Autodesk Inventor part; units mm, degrees
ref_plane "Work Plane1" through (29, 0, 0) normal (0, -1, 0) x (1, 0, 0)
ref_plane "YZ Plane" through (0, 0, 0) normal (1, 0, 0) x (0, 1, 0)
ref_plane "XZ Plane" through (0, 0, 0) normal (0, 1, 0) x (-1, 0, 0)
sketch "Sketch1" plane through (0, 0, 0) normal (0, 0, 1) x (1, 0, 0)
  line L0 (-0.0667, 0) -> (16, 0)
  line L1 (16, 0) -> (16, 2)
  line L2 (16, 2) -> (2.1, 2)
  line L3 (2.1, 2) -> (1.6705, 2)
  line L4 (1.6705, 2) -> (0, 2)
  line L5 (0, 2) -> (0, 3.8)
  line L6 (0, 3.8) -> (-2.2, 3.8)
  line L7 (-2.2, 3.8) -> (-2.2, 1.4434)
  line L8 (-2.2, 1.4434) -> (-0.9, 1.4434)
  line L9 (-0.9, 1.4434) -> (-0.0667, 0)
  line L10 (-5.84, 0) -> (19.64, 0)
  line L11 (0, -0.76) -> (0, 4.56)
  line L12 (2.1, 2) -> (0, 2) construction
  dimension "d1" = 13.9
  dimension "d2" = 0.4295
  dimension "d3" = 2.2
  dimension "d4" = 1.3
  dimension "d5" = 60
  dimension "d6" = 4
  dimension "d7" = 4
  dimension "d8" = 2.8868
  dimension "d9" = 7.6
  dimension "d26" = 16
revolve "Body" add sketch "Sketch1" angle 360 about axis through (-0.0667, 0, 0) along (1, 0, 0)
sketch "Sketch2" plane through (-2.2, 0, 0) normal (-1, 0, 0) x (0, 0, 1)
  circle A0 centre (0, 0) radius 1.4434
  line L0 (0, -5.32) -> (0, 5.32)
  line L1 (-5.32, 0) -> (5.32, 0)
  line L2 (1.4434, 0) -> (0.7217, -1.25)
  line L3 (0.7217, -1.25) -> (-0.7217, -1.25)
  line L4 (-0.7217, -1.25) -> (-1.4434, 0)
  line L5 (-1.4434, 0) -> (-0.7217, 1.25)
  line L6 (-0.7217, 1.25) -> (0.7217, 1.25)
  line L7 (0.7217, 1.25) -> (1.4434, 0)
  point P0 (0, 0)
extrude "Slot" add sketch "Sketch2" against normal up to next contours L7 A0 | A0 L2 | L6 L0 A0 | A0 L0 L3 | L0 L6 A0 | A0 L3 L0 | L4 A0 | A0 L5
fillet "Fillet1" radius 1.9 1 edges at (-2.2, -3.8, 0)
thread "Thread"
chamfer "Chamfer1" distance 0.4294 distance2 0.4294 1 edges at (16, -2, 0) measured on face at (16, 0.527, -0.2661)
ref_plane "Work Plane1" through (29, 0, 0) normal (0, -1, 0) x (1, 0, 0)
fillet "Fillet2" radius 0.4 1 edges at (0, -2, 0)
equation "\"d1\" = GEL"
equation "\"d3\" = KOH"
equation "\"d4\" = INTI"
equation "\"d6\" = GD"
equation "\"d7\" = BDM"
equation "\"d8\" = 1.1547 * SW"
equation "\"d9\" = KOD"
equation "\"d26\" = NLG"
equation "\"d30\" = R"
equation "\"d17\" = RR"
equation "\"d13\" = GEL"
equation "\"d15\" = -0.5 * SPD + 0.5 * GD"
equation "\"d16\" = GUL"
equation "\"GD\" = NND"
equation "\"NLG\" = 16"
equation "\"GEL\" = 13.9"
equation "\"KOD\" = 7.6"
equation "\"KOH\" = 2.2"
equation "\"INTI\" = 1.3"
equation "\"GAL\" = 0.61345 * PTC"
equation "\"GUL\" = 0.61345 * PTC"
equation "\"BDM\" = NND"
equation "\"SW\" = 2.5"
equation "\"RR\" = 1.9"
equation "\"SPD\" = NND - 1.2269 * PTC"
equation "\"R\" = 0.4"
equation "\"TOA\" = 30deg"
equation "\"GD1\" = THREADDIA - 1.2269 * PTC"
equation "\"THREADDIA\" = 4"
equation "\"PTC\" = 0.7"
equation "\"NND\" = 4"
equation "\"KOH1\" = 0.3"
equation "\"E0\" = 2.873"
properties part number "ISO 7380-1 - M4 x 16" material "Steel"
Build history of the part. All positions in model axes, mm. A direction names the side the tool comes from. Coordinates: 2 decimals unless noted, no trailing zeros. Order: outer loops, then holes, each group sorted by start corner. A loop starts at its lowest first (then second) coordinate and runs counter-clockwise, first axis right, second up. Notation, with made-up numbers: M 86,62.5 L 137,62.5 A15 ccw 137,69.5 Z; hole C 75.5,22.25 d3. An arc over 180 degrees is marked long. One line per question, with ' | ' between items. Start each with the question number.
1. Wall check: line 1 along X through (y, z) = (-1, -0.75); line 2 along X through (y, z) = (2.5, -1.5); line 3 along Z through (x, y) = (7, 1.75). Give the ranges that are in metal, low to high. Write a range as [from, to].
2. Cut at A-A (x = 8.75). Write the cut outline in (y, z), plus the area to 3 significant figures.
3. Mould opens along Z. For faces 3 (the face through (-1.5, 0.63, 1.08)), 4 (the face through (8, 0, 2)), 5 (the face through (0, 2.5, -0.8)) say: +Z half, -Z half, draft (parallel to the pull), parting line (faces both ways), or undercut.
4. Flat gauge pins, fed straight in: P1, Ø3, axis at x = 8, y = 0.5, coming from the -Z side; P2, Ø2, axis at y = -3, z = -1, coming from the +X side; P3, Ø1.1, axis at x = -1.5, z = 0, coming from the +Y side. Where does each tip first touch, or does it go through?
5. Tool access for faces 1 (the face through (-2, 1.25, 0)), 2 (the face through (-0.15, -2.8, -2.57)): list every direction of +Z, -Z, +X, -X, +Y, -Y with a clear straight run to the whole face (end or side of a thin tool).
The answers:
1) line 1: x = [-0.79, 16] | line 2: x = [-1.91, 0] | line 3: z = [-0.97, 0.97]
2) outline: C 0,0 d4 | area: 12.6 mm2
3) face 3: undercut | face 4: parting line | face 5: draft
4) P1: stops at z = -2 | P2: stops at x = 0.08 | P3: stops at y = 3.69
5) face 1: -X | face 2: +X, -X
